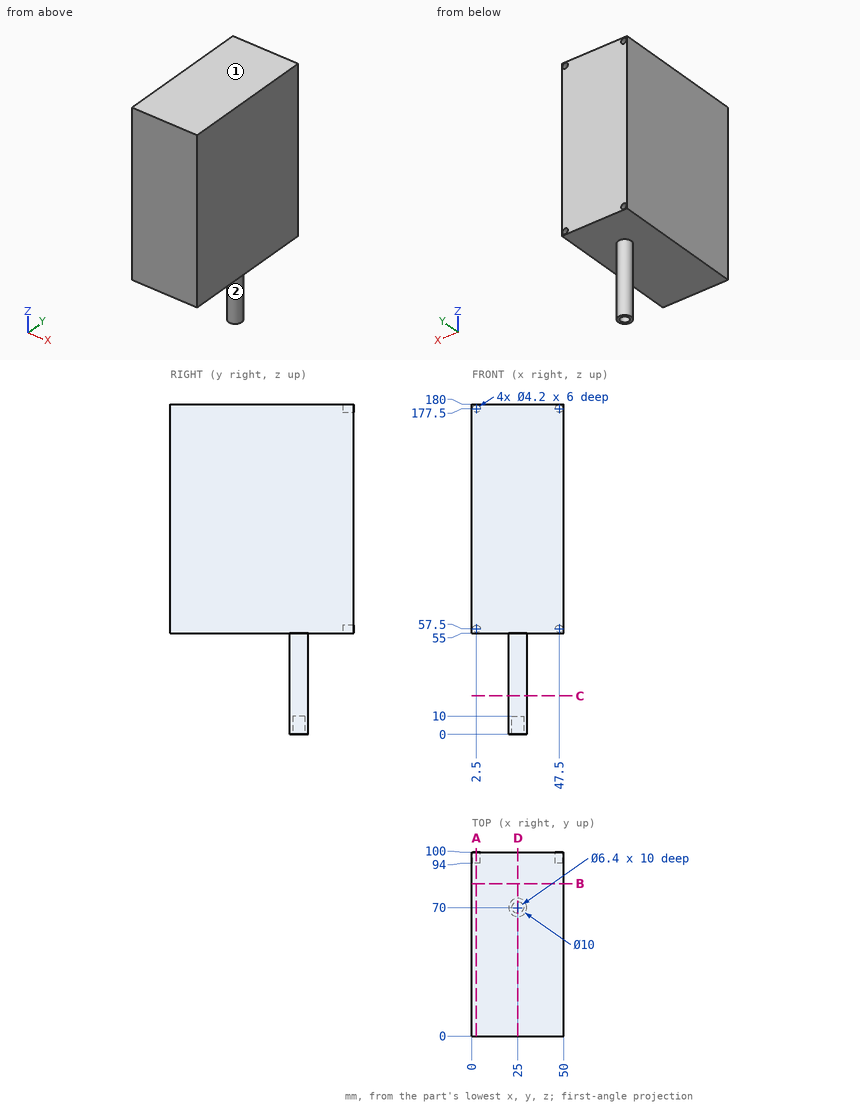
The figure shows three views and two pictorial views of one solid part (mm, origin at its lowest corner). Answer the questions. A direction names the side the tool comes from. Round coordinates to 2 decimals unless told otherwise and drop trailing zeros. Write each loop counter-clockwise with the first axis right and the second up, starting at its lowest first coordinate (ties: lowest second). Pieces come first, ordered by that corner, then holes. Notation, with made-up numbers: M -25,23 L -2,23 A10 ccw -2,32 Z; hole C 84.25,-4.5 d10. An arc over 180 degrees is marked long. Use a Markdown table: item, result.
1) The part is cut by section B-B (y = 83). Write down the section's boundary in (x, z), plus the area to 3 significant figures.
Answers follow:
| item | result |
|---|---|
| outline | M 0,55 L 50,55 L 50,180 L 0,180 Z |
| area | 6,250 mm2 |
2) The part is cut by section A-A (x = 2.5). Write down the section's boundary in (y, z), plus the area to 3 significant figures.
Answers follow:
| item | result |
|---|---|
| outline | M 0,55 L 100,55 L 100,55.4 L 94,55.4 L 94,59.6 L 100,59.6 L 100,175.4 L 94,175.4 L 94,179.6 L 100,179.6 L 100,180 L 0,180 Z |
| area | 12,400 mm2 |
3) Flat-ended cylindrical pins translate along their axes: pin 1 (5 mm diameter, centred on x = 47.5, z = 177.5, fed in from +Y); pin 2 (2 mm diameter, centred on x = 47.5, z = 57.5, fed in from +Y); pin 3 (8 mm diameter, centred on x = 20, y = 78, fed in from -Z); pin 4 (1.9 mm diameter, centred on x = 24.5, y = 69, fed in from -Z). Find the tip coordinate at first contact, or state that the pin passes through.
Answers follow:
| item | result |
|---|---|
| pin 1 | stops at y = 100 |
| pin 2 | stops at y = 94 |
| pin 3 | stops at z = 55 |
| pin 4 | stops at z = 10 |
4) The part is cut by section D-D (x = 25). Write down the section's boundary in (y, z), plus the area to 3 significant figures.
Answers follow:
| item | result |
|---|---|
| outline | M 0,55 L 65,55 L 65,0 L 66.8,0 L 66.8,10 L 73.2,10 L 73.2,0 L 75,0 L 75,55 L 100,55 L 100,180 L 0,180 Z |
| area | 13,000 mm2 |
5) Straight lines are drawn through the part: line 1 along X through (y, z) = (97.65, 57.5); line 2 along Y through (x, z) = (25, 2); line 3 along X through (y, z) = (97, 177). For each, find the intervals that lie inside material, in ascending order. Write a range as [from, to].
Answers follow:
| item | result |
|---|---|
| line 1 | x = [0, 0.4], [4.6, 45.4], [49.6, 50] |
| line 2 | y = [65, 66.8], [73.2, 75] |
| line 3 | x = [0, 0.46], [4.54, 45.46], [49.54, 50] |
6) A tool of negligible diameter and unlimited length cuts with its end or side. For the marked faces 1 and 2, from which of +Z, -Z, +X, -X, +Y, -Y can it reach the whole face along a straight path? Write none if from no direction.
Answers follow:
| item | result |
|---|---|
| face 1 | +Z, +X, -X, +Y, -Y |
| face 2 | -Z |
7) The part is cut by section C-C (z = 21). Write down the section's boundary in (x, y), plus the area to 3 significant figures.
Answers follow:
| item | result |
|---|---|
| outline | C 25,70 d10 |
| area | 78.5 mm2 |
